Input: part model. Units: mm. Frame: model coordinates. Face numbers are marked on the shaded views. A direction names the side the tool comes from. Give positions to 0.01 mm unless a question says otherwise; leave off trailing zeros. Loops run counter-clockwise (first coordinate to the right, second up) from the corner with the lowest first, then second, coordinate; pieces in that order, holes last.
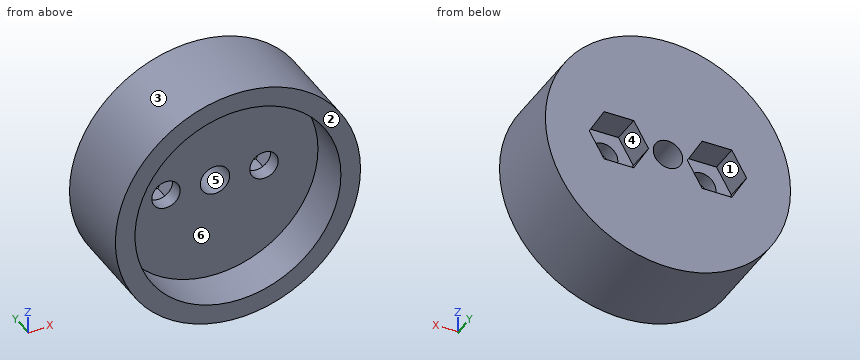
from build123d import *

# Parameters (mm, degrees)
F0_R     = 10.5
F0_R_2   = 1.5
F1_DEPTH = 4.5
F0_R_3   = 12.5
F2_DEPTH = 9
F4_DEPTH = 4.5
F3_R     = 1.45
F5_DEPTH = 4.5
F6_DEPTH = 3


with BuildPart() as f1:
    # F0 (on Front) → F1 (new body)
    with BuildSketch(Plane.XZ):
        Circle(F0_R)
        Circle(F0_R_2, mode=Mode.SUBTRACT)
    extrude(amount=F1_DEPTH)

    # F0 (on Front) → F2 (join)
    with BuildSketch(Plane.XZ):
        Circle(F0_R_3)
        Circle(F0_R, mode=Mode.SUBTRACT)
    extrude(amount=F2_DEPTH)

    # F3 (on face) → F4 (cut)
    with BuildSketch(Plane(origin=(0, 0, 0), x_dir=(-1, 0, 0), z_dir=(0, 1, 0))):
        with BuildLine():
            ThreePointArc((6.45, 0), (5, 1.45), (3.55, 0))
            ThreePointArc((3.55, 0), (5, -1.45), (6.45, 0))
        make_face()
    extrude(amount=-F4_DEPTH, mode=Mode.SUBTRACT)

    # F3 (on face) → F5 (cut)
    with BuildSketch(Plane(origin=(0, 0, 0), x_dir=(-1, 0, 0), z_dir=(0, 1, 0))):
        with Locations((-5, 0)):
            Circle(F3_R)
    extrude(amount=-F5_DEPTH, mode=Mode.SUBTRACT)

    # F3 (on face) → F6 (cut)
    with BuildSketch(Plane(origin=(0, 0, 0), x_dir=(-1, 0, 0), z_dir=(0, 1, 0))):
        Polygon((-1.975, 0), (-3.4875, 2.619727), (-6.5125, 2.619727), (-8.025, 0), (-6.5125, -2.619727), (-3.4875, -2.619727), align=None)
        with Locations((-5, 0)):
            Circle(F3_R, mode=Mode.SUBTRACT)
        Polygon((3.4875, 2.619727), (1.975, 0), (3.4875, -2.619727), (6.5125, -2.619727), (8.025, 0), (6.5125, 2.619727), align=None)
        with BuildLine():
            ThreePointArc((6.45, 0), (5, -1.45), (3.55, 0))
            ThreePointArc((3.55, 0), (5, 1.45), (6.45, 0))
        make_face(mode=Mode.SUBTRACT)
    extrude(amount=-F6_DEPTH, mode=Mode.SUBTRACT)


solid = f1.part
(1) Mould query, pull axis X, two halves, no side actions, for the marked faces 1, 2 and 3. Classes: +X half, -X half, draft (parallel to the pull), parting line (faces both ways), or undercut.
Values follow:
face 1: undercut
face 2: draft
face 3: parting line
(2) Cut plane D-D (x = 9.75). Return the cut outline in (y, z).
Values follow:
outline: (-9, -7.82) - (0, -7.82) - (0, 7.82) - (-9, 7.82) - (-9, 3.9) - (-4.5, 3.9) - (-4.5, -3.9) - (-9, -3.9) - close
(3) Pin query (flat end, axial travel): pin 1 Ø5 at (x, y) = (3, -4) entering from -Z; pin 2 Ø4 at (x, z) = (1.5, -4) entering from +Y; pin 3 Ø2.5 at (x, y) = (-5.5, -1.5) entering from -Z; pin 4 Ø2 at (x, z) = (-2.5, -8) entering from -Y. Return the tip coordinate at first contact, or that it passes through.
Values follow:
pin 1: stops at z = -12.49
pin 2: stops at y = 0
pin 3: stops at z = -11.76
pin 4: stops at y = -4.5
(4) Cut plane B-B (y = -1.25). Return the cut outline in (x, z) (1 decimal), and give its area (3 significant figures).
Values follow:
outline: circle Ø25 at (0, 0); hole (-8, 0) - (-6.5, -2.6) - (-3.5, -2.6) - (-2, 0) - (-3.5, 2.6) - (-6.5, 2.6) - close; hole circle Ø3 at (0, 0); hole (2, 0) - (3.5, -2.6) - (6.5, -2.6) - (8, 0) - (6.5, 2.6) - (3.5, 2.6) - close
area: 436 mm2
(5) Cut plane A-A (x = 0). Return the cut outline in (y, z), and give its area (3 significant figures).
Values follow:
outline: (-9, -12.5) - (0, -12.5) - (0, -1.5) - (-4.5, -1.5) - (-4.5, -10.5) - (-9, -10.5) - close; (-9, 10.5) - (-4.5, 10.5) - (-4.5, 1.5) - (0, 1.5) - (0, 12.5) - (-9, 12.5) - close
area: 117 mm2
(6) Reachability of the marked faces 4, 5 and 6 from +Z, -Z, +X, -X, +Y, -Y: full face, straight path, thin tool, end or side. Return the list, or none.
Values follow:
face 4: +Y
face 5: +Y, -Y
face 6: -Y
(7) Ray query, probe 1 along Z at (x, y) = (0, -6.15); probe 2 along Z at (x, y) = (0, -2.1); probe 3 along X at (y, z) = (-6.5, 0.5). Return the intervals inside material, ascending.
Values follow:
probe 1: z = -12.5 to -10.5, 10.5 to 12.5
probe 2: z = -12.5 to -1.5, 1.5 to 12.5
probe 3: x = -12.49 to -10.49, 10.49 to 12.49
(8) Cut plane C-C (z = -0.5). Return the cut outline in (x, y).
Values follow:
outline: (-12.49, -9) - (-10.49, -9) - (-10.49, -4.5) - (-6.36, -4.5) - (-6.36, -3) - (-7.74, -3) - (-7.74, 0) - (-12.49, 0) - close; (-3.64, -4.5) - (-1.41, -4.5) - (-1.41, 0) - (-2.26, 0) - (-2.26, -3) - (-3.64, -3) - close; (1.41, -4.5) - (3.64, -4.5) - (3.64, -3) - (2.26, -3) - (2.26, 0) - (1.41, 0) - close; (6.36, -4.5) - (10.49, -4.5) - (10.49, -9) - (12.49, -9) - (12.49, 0) - (7.74, 0) - (7.74, -3) - (6.36, -3) - close
